```python
from build123d import *

# Parameters (mm, degrees)
F1_W     = 90.75
F1_H     = 149
F1_W_2   = 84.75
F1_H_2   = 143
F2_DEPTH = 44.5
F3_DEPTH = 2
F4_SIZE  = 2
F5_W     = 88.35
F5_H     = 146.6
F6_DEPTH = 3
F7_W     = 90.75
F7_H     = 149
F7_W_2   = 87.75
F7_H_2   = 146
F8_DEPTH = 2.5


with BuildPart() as f2:
    # F1 (on Top) → F2 (new body)
    with BuildSketch(Plane.XY):
        Rectangle(F1_W, F1_H)
        Rectangle(F1_W_2, F1_H_2, mode=Mode.SUBTRACT)
    extrude(amount=F2_DEPTH)

    # F1 (on Top) → F3 (join)
    with BuildSketch(Plane.XY):
        Rectangle(F1_W, F1_H)
        Rectangle(F1_W_2, F1_H_2, mode=Mode.SUBTRACT)
        Rectangle(F1_W_2, F1_H_2)
    extrude(amount=F3_DEPTH)

    # F4
    f4_edges = [f2.edges().sort_by_distance(p)[0] for p in [
        (0, 71.5, 2),
        (42.375, 0, 2),
        (-42.375, 0, 2),
        (0, -71.5, 2),
        (42.375, -71.5, 23.25),
        (42.375, 71.5, 23.25),
        (-42.375, 71.5, 23.25),
        (-42.375, -71.5, 23.25),
    ]]
    chamfer(f4_edges, length=F4_SIZE)

    # F5 (on face) → F6 (cut)
    with BuildSketch(Plane.XY.offset(44.5)):
        Rectangle(F5_W, F5_H)
        Polygon((-40.375, -71.5), (-42.375, -69.5), (-42.375, 69.5), (-40.375, 71.5), (40.375, 71.5), (42.375, 69.5), (42.375, -69.5), (40.375, -71.5), align=None, mode=Mode.SUBTRACT)
    extrude(amount=-F6_DEPTH, mode=Mode.SUBTRACT)

    # F7 (on face) → F8 (cut)
    with BuildSketch(Plane(origin=(0, 0, 0), x_dir=(1, 0, 0), z_dir=(0, 0, -1))):
        Rectangle(F7_W, F7_H)
        Rectangle(F7_W_2, F7_H_2, mode=Mode.SUBTRACT)
    extrude(amount=-F8_DEPTH, mode=Mode.SUBTRACT)


solid = f2.part
```
Verification items for the finished model (mm, model axes). A direction names the side the tool comes from. Give positions to 0.01 mm unless a question says otherwise; leave off trailing zeros. Write each loop counter-clockwise with the first axis right and the second up, starting at its lowest first coordinate (ties: lowest second). Pieces come first, ordered by that corner, then holes. Notation, with made-up numbers: (-21, 61) - (4, 61) arc R12 ccw to (4, 70) - close; hole circle Ø9 at (-39.5, 33). An arc over 180 degrees is marked (long way). Put each result on its own line as item: value.
Q1. Depth check by flat-ended pin: P1, Ø12, axis at x = 11, y = 42, coming from the +Z side. Enter the tip coordinate at first touch or a pass-through.
Result:
P1: z = 2
Q2. Set-up check for faces 4 (the face through (45.375, -1, 23)), 5 (the face through (42.375, -1, 22)): record each of +Z, -Z, +X, -X, +Y, -Y from which the full face is reachable in a straight line by a thin tool's end or side.
Result:
face 4: +Z, -Z, +X, +Y, -Y
face 5: +Z
Q3. Mould release check, pull along Y, two halves, no side actions. Record for faces 1 (the face through (-1, 74.5, 23)), 2 (the face through (-45.375, -1, 23)), 3 (the face through (-1, 73.3, 43)): released by +Y, released by -Y, zero draft, split by the parting line, or undercut.
Result:
face 1: released by +Y
face 2: zero draft
face 3: undercut
Q4. Section check C-C on x = 24. Record the cut outline in (y, z).
Result:
outline: (-74.5, 2.5) - (-73, 2.5) - (-73, 0) - (73, 0) - (73, 2.5) - (74.5, 2.5) - (74.5, 44.5) - (73.3, 44.5) - (73.3, 41.5) - (71.5, 41.5) - (71.5, 4) - (69.5, 2) - (-69.5, 2) - (-71.5, 4) - (-71.5, 41.5) - (-73.3, 41.5) - (-73.3, 44.5) - (-74.5, 44.5) - close
Q5. Section check A-A on z = 23. Record the cut outline in (x, y) (3 decimals), and give its area (3 significant figures).
Result:
outline: (-45.375, -74.5) - (45.375, -74.5) - (45.375, 74.5) - (-45.375, 74.5) - close; hole (-42.375, -69.5) - (-40.375, -71.5) - (40.375, -71.5) - (42.375, -69.5) - (42.375, 69.5) - (40.375, 71.5) - (-40.375, 71.5) - (-42.375, 69.5) - close
area: 1,410 mm2
Q6. Section check B-B on y = 54. Record the cut outline in (x, z) (3 decimals), and give its area (3 significant figures).
Result:
outline: (-45.375, 2.5) - (-43.875, 2.5) - (-43.875, 0) - (43.875, 0) - (43.875, 2.5) - (45.375, 2.5) - (45.375, 44.5) - (44.175, 44.5) - (44.175, 41.5) - (42.375, 41.5) - (42.375, 4) - (40.375, 2) - (-40.375, 2) - (-42.375, 4) - (-42.375, 41.5) - (-44.175, 41.5) - (-44.175, 44.5) - (-45.375, 44.5) - close
area: 422 mm2
Q7. Scan lines: probe 1 along Y at (x, z) = (-17, 29.5); probe 2 along X at (y, z) = (-64, 33) (3 decimals); probe 3 along X at (y, z) = (-32, 42) (3 decimals). Record each from-to range of solid material in increasing order. Write a range as from..to.
Result:
probe 1: -74.5..-71.5, 71.5..74.5
probe 2: -45.375..-42.375, 42.375..45.375
probe 3: -45.375..-44.175, 44.175..45.375
